Work out the finished part from the listing and answer in its coordinate system (mm). A direction names the side the tool comes from. Give positions to 0.01 mm unless a question says otherwise; leave off trailing zeros. Order: outer loops, then holes, each group sorted by start corner. A loop starts at its lowest first (then second) coordinate and runs counter-clockwise, first axis right, second up.
```python
from build123d import *

# Parameters (mm, degrees)
F0_W      = 271.8892842531
F0_H      = 97.4458288401
F1_DEPTH  = 101.6
F3_R      = 5.08
F4_W      = 16.6076868773
F4_H      = 76.0046169162
F5_DEPTH  = 107.696
F6_W      = 15.0446221232
F6_H      = 74.8323127627
F7_DEPTH  = 107.696
F2_W      = 236.4497035742
F2_H      = 73.7357586622
F8_DEPTH  = 77.978
F9_W      = 139.5306698978
F9_H      = 149.727134034
F10_DEPTH = 131.318
F11_R     = 12.7
F12_W     = 30.5456686765
F12_H     = 35.9262302518
F13_DEPTH = 127
F15_DEPTH = 65.278
F17_DEPTH = 70.104
F18_R     = 6.7219361341
F19_DEPTH = 40.894
F21_DEPTH = 100.584
F22_R     = 6.0147460443
F23_DEPTH = 25.4
F24_R     = 5.08
F25_R     = 8.5849434278


with BuildPart() as f1:
    # F0 (on Top) → F1 (new body)
    with BuildSketch(Plane.XY):
        with Locations((10.5727538466, -18.0099094287)):
            Rectangle(F0_W, F0_H)
    extrude(amount=F1_DEPTH)

    # F3
    f3_edges = [f1.edges().sort_by_distance(p)[0] for p in [
        (-125.371888, -66.732824, 50.8),
        (146.517396, -66.732824, 50.8),
        (10.572754, -66.732824, 0),
        (10.572754, -66.732824, 101.6),
        (146.517396, 30.713005, 50.8),
        (146.517396, -18.009909, 0),
        (146.517396, -18.009909, 101.6),
        (-125.371888, 30.713005, 50.8),
        (10.572754, 30.713005, 0),
        (10.572754, 30.713005, 101.6),
        (-125.371888, -18.009909, 0),
        (-125.371888, -18.009909, 101.6),
    ]]
    fillet(f3_edges, radius=F3_R)

    # F4 (on face) → F5 (join)
    with BuildSketch(Plane(origin=(0, 0, 0), x_dir=(1, 0, 0), z_dir=(0, 0, -1))):
        with Locations((-101.2849360704, 17.3892304301)):
            Rectangle(F4_W, F4_H)
    extrude(amount=F5_DEPTH)

    # F6 (on face) → F7 (join)
    with BuildSketch(Plane(origin=(0, 0, 0), x_dir=(1, 0, 0), z_dir=(0, 0, -1))):
        with Locations((122.6258315146, 16.998462379)):
            Rectangle(F6_W, F6_H)
    extrude(amount=F7_DEPTH)

    # F2 (on face) → F8 (cut)
    with BuildSketch(Plane.XY.offset(101.6)):
        with Locations((9.42825526, -17.3080377281)):
            Rectangle(F2_W, F2_H)
    extrude(amount=-F8_DEPTH, mode=Mode.SUBTRACT)

    # F9 (on face) → F10 (join)
    with BuildSketch(Plane.YZ.offset(146.5173959732)):
        with Locations((-14.6516356617, 49.1371015087)):
            Rectangle(F9_W, F9_H)
    extrude(amount=F10_DEPTH)

    # F11
    f11_edges = [f1.edges().sort_by_distance(p)[0] for p in [
        (212.176396, 55.113699, 124.000669),
        (212.176396, -84.416971, 124.000669),
        (146.517396, -14.651636, 124.000669),
        (277.835396, -14.651636, 124.000669),
        (212.176396, -84.416971, -25.726466),
        (146.517396, -84.416971, 49.137102),
        (277.835396, -84.416971, 49.137102),
        (277.835396, -14.651636, -25.726466),
        (277.835396, 55.113699, 49.137102),
        (212.176396, 55.113699, -25.726466),
        (146.517396, 55.113699, 49.137102),
        (146.517396, -14.651636, -25.726466),
    ]]
    fillet(f11_edges, radius=F11_R)

    # F12 (on face) → F13 (join)
    with BuildSketch(Plane.YZ.offset(277.8353959732)):
        with Locations((-15.2728343382, 17.9631151259)):
            Rectangle(F12_W, F12_H)
    extrude(amount=F13_DEPTH)

    # F14 (on face) → F15 (join)
    with BuildSketch(Plane.XZ.offset(84.4169706106)):
        Polygon((166.5966212749, 103.4740507603), (163.0362123251, 104.4450700283), (163.0362123251, 30.6476131082), (166.5966212749, 30.6476131082), align=None)
    extrude(amount=F15_DEPTH)

    # F16 (on face) → F17 (join)
    with BuildSketch(Plane(origin=(0, 55.1136992872, 0), x_dir=(-1, 0, 0), z_dir=(0, 1, 0))):
        Polygon((-165.8086842582, 36.9507782161), (-165.3019338846, 103.3622100949), (-169.9908971786, 103.3622100949), (-169.9908971786, 36.9507782161), align=None)
    extrude(amount=F17_DEPTH)

    # F18 (on face) → F19 (join)
    with BuildSketch(Plane.YZ.offset(277.8353959732)):
        with Locations((-48.636149615, 15.0712924078)):
            Circle(F18_R)
        with Locations((15.748, 15.494)):
            Circle(F18_R)
    extrude(amount=F19_DEPTH)

    # F20 (on face) → F21 (join)
    with BuildSketch(Plane(origin=(-125.3718882799, 0, 0), x_dir=(0, -1, 0), z_dir=(-1, 0, 0))):
        Polygon((23.6901119351, 83.874464035), (17.8975313902, 88.5533466935), (17.8975313902, 83.874464035), align=None)
    extrude(amount=F21_DEPTH)

    # F22 (on face) → F23 (cut)
    with BuildSketch(Plane.YZ.offset(277.8353959732)):
        with Locations((-50.5576916039, 72.7600604296)):
            Circle(F22_R)
        with Locations((21.8323083961, 72.7600604296)):
            Circle(F22_R)
    extrude(amount=-F23_DEPTH, mode=Mode.SUBTRACT)

    # F24
    f24_edges = [f1.edges().sort_by_distance(p)[0] for p in [
        (318.729396, -55.358086, 15.071292),
        (318.729396, 9.026064, 15.494),
    ]]
    fillet(f24_edges, radius=F24_R)

    # F25
    f25_edges = [f1.edges().sort_by_distance(p)[0] for p in [
        (404.835396, -15.272834, 35.92623),
        (404.835396, -30.545669, 17.963115),
        (404.835396, -15.272834, 0),
        (404.835396, 0, 17.963115),
    ]]
    fillet(f25_edges, radius=F25_R)


solid = f1.part
```
1. The part is cut by section C-C (y = -91). Write down the section's boundary in (x, z), then the cut area to 3 significant figures.
Findings below:
outline: (163.04, 30.65) - (166.6, 30.65) - (166.6, 103.47) - (163.04, 104.45) - close
area: 261 mm2
2. The part is cut by section A-A (z = -63). Write down the section's boundary in (x, y), then the cut area to 3 significant figures.
Findings below:
outline: (-109.59, -55.39) - (-92.98, -55.39) - (-92.98, 20.61) - (-109.59, 20.61) - close; (115.1, -54.41) - (130.15, -54.41) - (130.15, 20.42) - (115.1, 20.42) - close
area: 2,390 mm2
3. The part is cut by section B-B (x = 51.5). Write down the section's boundary in (y, z).
Findings below:
outline: (-66.73, 5.08) arc R5.08 ccw to (-61.65, 0) - (25.63, 0) arc R5.08 ccw to (30.71, 5.08) - (30.71, 96.52) arc R5.08 ccw to (25.63, 101.6) - (19.56, 101.6) - (19.56, 23.62) - (-54.18, 23.62) - (-54.18, 101.6) - (-61.65, 101.6) arc R5.08 ccw to (-66.73, 96.52) - close
4. Straight lines are drawn through the part: probe 1 along X at (y, z) = (-11, 63.5); probe 2 along Y at (x, z) = (126.5, 55); probe 3 along X at (y, z) = (-7.5, -24). For each, find the intervals that lie inside material, in ascending order.
Findings below:
probe 1: x = -125.37 to -108.8, 127.65 to 277.84
probe 2: y = -66.73 to -54.18, 19.56 to 30.71
probe 3: x = -109.59 to -92.98, 115.1 to 130.15, 152.82 to 271.53
5. The part is cut by section D-D (x = -141.5). Write down the section's boundary in (y, z), then the cut area to 3 significant figures.
Findings below:
outline: (-23.69, 83.87) - (-17.9, 83.87) - (-17.9, 88.55) - close
area: 13.6 mm2
6. Which of the six approach directions +Z, -Z, +X, -X, +Y, -Y give full straight-line access (tool end or side, diameter ignored) to faces 1 (the face through (130.148, -16, -53)), 2 (the face through (8, -17, 23.622)), 3 (the face through (-101, 20.613, -53)), 4 (the face through (336, -15, 0)), 5 (the face through (252.435, -51, 73))?
Findings below:
face 1: -Z, +Y, -Y
face 2: +Z
face 3: -Z, -X, +Y
face 4: -Z, +X, +Y, -Y
face 5: +X
7. Given P1, Ø22, axis at y = -33.5, z = 45, coming from the -X side; P2, Ø12, axis at x = 246.5, z = 6.5, coming from the +Y side; P3, Ø15.5, axis at x = 332.5, y = -14.5, coming from the -Z side, each flat-ended and moving along its own axis, determine where each tip first touches the part or whether it passes through.
Findings below:
P1: stops at x = -125.37
P2: stops at y = 55.11
P3: stops at z = 0
8. The mould has two halves that part along X. Classify faces 6 (the face through (404.835, -15, 18)), 7 (the face through (265.31, -44.82, 74.57)), 8 (the face through (115.104, -16, -53)): pulls with the +X half, pulls with the -X half, needs draft (parallel to the pull), parting line crosses it, or undercut.
Findings below:
face 6: pulls with the +X half
face 7: needs draft
face 8: undercut
